Answer from the drawing. Dimensions are ordinates in mm from the lowest x, y and z of the part. A direction names the side the tool comes from. Give positions to 0.01 mm unless a question says otherwise; leave off trailing zeros. Loops run counter-clockwise (first coordinate to the right, second up) from the corner with the lowest first, then second, coordinate; pieces in that order, holes last. Notation, with made-up numbers: (33.5, -8) -> (91.5, -8) arc R13 cw to (91.5, 1) -> close; hole circle Ø11 at (80.25, 80). An arc over 180 degrees is marked (long way). Answer as CSV lines item,"result". Start each with the question number.
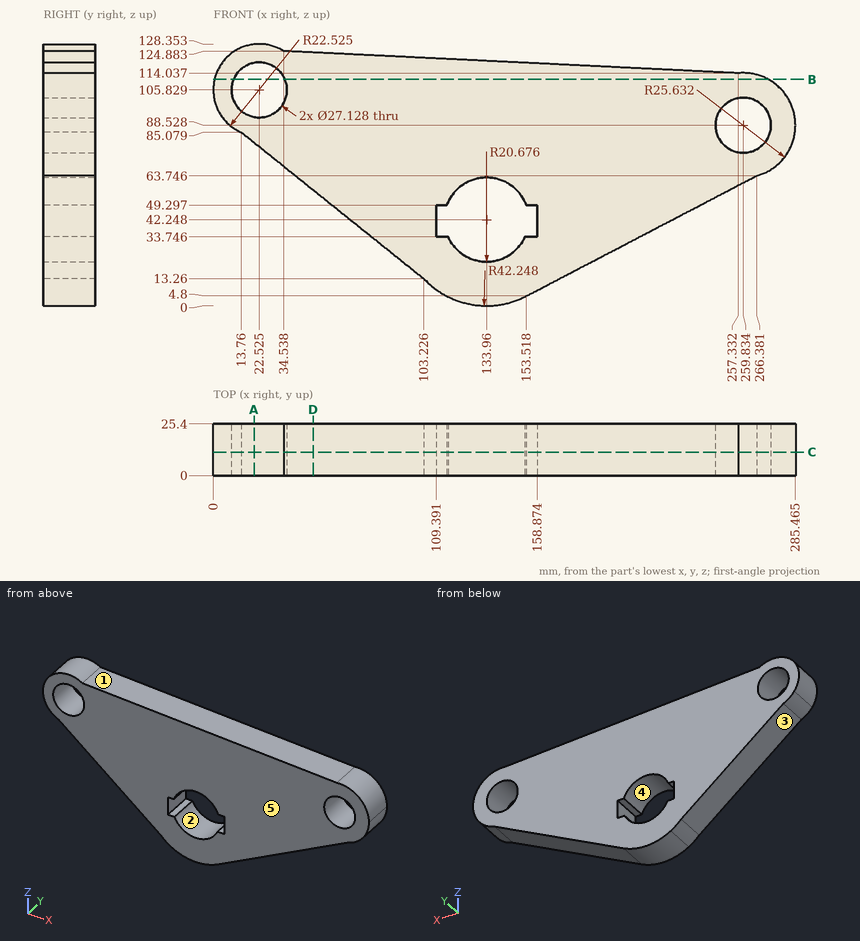
(1) A tool of negligible diameter and unlimited length cuts with its end or side. For the marked faces 1 and 2, from which of +Z, -Z, +X, -X, +Y, -Y can it reach the whole face along a straight path? Write none if from no direction.
(2) Find section A-A on x = 20. Write down the section's boundary in (y, z) (1 decimal), then the cut area to 3 significant figures.
(3) Find section C-C on y = 11.5. Give the number of separate pieces and of enclosed holes in the cut face, then the cut area to 3 significant figures.
(4) Each of these flat-tipped pins is pushed along its axis until it touches: P1, Ø12.5, axis at y = 12, z = 45, coming from the +X side (1 decimal); P2, Ø2, axis at x = 130, y = 11.5, coming from the -Z side; P3, Ø1.6, axis at x = 155, y = 8.5, coming from the -Z side (1 decimal); P4, Ø12, axis at x = 251, z = 42.5, coming from the -Y side. Where does it stop, or does it pass through?
(5) Find section B-B on z = 111. Write down the section's boundary in (x, y) (1 decimal).
(6) Find the intervals of material crossed by line 1 along X through (y, z) = (17.75, 97.5) (1 decimal); line 2 along X through (y, z) = (18.75, 99.5) (1 decimal); line 3 along X through (y, z) = (22.5, 87.5) (1 decimal), in increasing order. Write a range as from..to.
(7) The mould has two halves that part along X. Classify the marked faces 3, 4 and 5: pulls with the +X half, pulls with the -X half, needs draft (parallel to the pull), parting line crosses it, or undercut.
(8) Find section D-D on x = 49. Write down the section's boundary in (y, z), then the cut area to 3 significant figures.
Answer block:
1,face 1,"+Z, +X, +Y, -Y"
1,face 2,"+Y, -Y"
2,outline,"(0, 80.1) -> (25.4, 80.1) -> (25.4, 92.5) -> (0, 92.5) -> close; (0, 119.2) -> (25.4, 119.2) -> (25.4, 128.2) -> (0, 128.2) -> close"
2,area,"546 mm2"
3,separate pieces,"1"
3,enclosed holes,"3"
3,area,"20,300 mm2"
4,P1,"stops at x = 242.5"
4,P2,"stops at z = 0.1"
4,P3,"stops at z = 5.2"
4,P4,"passes through"
5,outline,"(0.6, 0) -> (10, 0) -> (10, 25.4) -> (0.6, 25.4) -> close; (35.1, 0) -> (272.2, 0) -> (272.2, 25.4) -> (35.1, 25.4) -> close"
6,line 1,"x = 1.6..11.8, 33.2..249.7, 270..283.8"
6,line 2,"x = 0.9..10.5, 34.5..251.9, 267.8..283"
6,line 3,"x = 9.4..246.3, 273.4..285.4"
7,face 3,"pulls with the -X half"
7,face 4,"undercut"
7,face 5,"needs draft"
8,outline,"(0, 56.79) -> (25.4, 56.79) -> (25.4, 124.18) -> (0, 124.18) -> close"
8,area,"1,710 mm2"
